from build123d import *

# Parameters (mm, degrees)
SKETCH1_R           = 87
SKETCH1_R_2         = 10
BOSS_EXTRUDE1_DEPTH = 5
SKETCH2_R           = 80
SKETCH2_R_2         = 76
BOSS_EXTRUDE2_DEPTH = 30
SKETCH3_R           = 87
SKETCH3_R_2         = 80
BOSS_EXTRUDE3_DEPTH = 20


with BuildPart() as part:
    # Sketch1 → Boss-Extrude1 (new body)
    with BuildSketch(Plane(origin=(0, 0, 0), x_dir=(1, 0, 0), z_dir=(0, 1, 0))):
        with Locations(Location((0, 0, 0), (0, 0, 270))):
            Circle(SKETCH1_R)
        with Locations(Location((0, 51.875, 0), (0, 0, 270))):
            Circle(SKETCH1_R_2, mode=Mode.SUBTRACT)
        with Locations(Location((44.926567821, -25.936633975, 0), (0, 0, 270))):
            Circle(SKETCH1_R_2, mode=Mode.SUBTRACT)
        with Locations(Location((-44.923567821, -25.938366025, 0), (0, 0, 270))):
            Circle(SKETCH1_R_2, mode=Mode.SUBTRACT)
    extrude(amount=BOSS_EXTRUDE1_DEPTH)

    # Sketch2 → Boss-Extrude2 (add)
    with BuildSketch(Plane(origin=(0, 5, 0), x_dir=(1, 0, 0), z_dir=(0, 1, 0))):
        with Locations(Location((0, 0, 0), (0, 0, 270))):
            Circle(SKETCH2_R)
        with Locations(Location((0, 0, 0), (0, 0, 270))):
            Circle(SKETCH2_R_2, mode=Mode.SUBTRACT)
    extrude(amount=BOSS_EXTRUDE2_DEPTH)

    # Sketch3 → Boss-Extrude3 (add)
    with BuildSketch(Plane(origin=(0, 5, 0), x_dir=(1, 0, 0), z_dir=(0, 1, 0))):
        with Locations(Location((0, 0, 0), (0, 0, 270))):
            Circle(SKETCH3_R)
        with Locations(Location((0, 0, 0), (0, 0, 270))):
            Circle(SKETCH3_R_2, mode=Mode.SUBTRACT)
    extrude(amount=BOSS_EXTRUDE3_DEPTH)


solid = part.part
Input: part model. Units: mm. Frame: model coordinates. A direction names the side the tool comes from. Round coordinates to 2 decimals unless told otherwise and drop trailing zeros. Order: outer loops, then holes, each group sorted by start corner. A loop starts at its lowest first (then second) coordinate and runs counter-clockwise, first axis right, second up. Notation, with made-up numbers: (14, -29) - (19, -29) arc R22 cw to (19, -21) - close; hole circle Ø8 at (9.5, 56). An arc over 180 degrees is marked (long way). Use a Markdown table: item, result.
1. Mould query, pull axis Z, two halves, no side actions, for faces 3 (the face through (-29, 35, 71)), 4 (the face through (-78.1, 29.93, -17.34)), 5 (the face through (36.055, 2.465, 30.551)). Classes: +Z half, -Z half, draft (parallel to the pull), parting line (faces both ways), or undercut.
Evaluation:
| item | result |
|---|---|
| face 3 | draft |
| face 4 | parting line |
| face 5 | undercut |
2. Material intervals for probe 1 along X at (y, z) = (23, -2.5); probe 2 along Z at (x, y) = (1.5, 28); probe 3 along Y at (x, z) = (70, 26), sorted ascending.
Evaluation:
| item | result |
|---|---|
| probe 1 | -86.96 to -75.96, 75.96 to 86.96 |
| probe 2 | -79.99 to -75.99, 75.99 to 79.99 |
| probe 3 | 0 to 5 |
3. Section B-B on z = 32. Return the cut outline in (x, y).
Evaluation:
| item | result |
|---|---|
| outline | (-80.9, 0) - (-52.88, 0) - (-52.88, 5) - (-68.93, 5) - (-68.93, 35) - (-73.32, 35) - (-73.32, 25) - (-80.9, 25) - close; (-36.97, 0) - (36.97, 0) - (36.97, 5) - (-36.97, 5) - close; (52.88, 0) - (80.9, 0) - (80.9, 25) - (73.32, 25) - (73.32, 35) - (68.93, 35) - (68.93, 5) - (52.88, 5) - close |
4. Section A-A on x = 0. Return the cut outline in (y, z) (3 decimals).
Evaluation:
| item | result |
|---|---|
| outline | (0, -87) - (25, -87) - (25, -80) - (35, -80) - (35, -76) - (5, -76) - (5, -61.875) - (0, -61.875) - close; (0, -41.875) - (5, -41.875) - (5, 76) - (35, 76) - (35, 80) - (25, 80) - (25, 87) - (0, 87) - close |
5. Section C-C on z = -59.5. Return the cut outline in (x, y), then the cut area to 3 significant figures.
Evaluation:
| item | result |
|---|---|
| outline | (-63.47, 0) - (-6.47, 0) - (-6.47, 5) - (-47.28, 5) - (-47.28, 35) - (-53.48, 35) - (-53.48, 25) - (-63.47, 25) - close; (6.47, 0) - (63.47, 0) - (63.47, 25) - (53.48, 25) - (53.48, 35) - (47.28, 35) - (47.28, 5) - (6.47, 5) - close |
| area | 1,340 mm^2 |
6. Access query for faces 1 (the face through (86.26, 12.32, -11.33)), 2 (the face through (1, 5, -1)). Directions: +Z, -Z, +X, -X, +Y, -Y. A direction counts if a zero-diameter tool reaches every point of the face in a straight line with its end or side. Return the directions, or none.
Evaluation:
| item | result |
|---|---|
| face 1 | +Y, -Y |
| face 2 | +Y |
7. Section D-D on y = 10.5. Return the cut outline in (x, z).
Evaluation:
| item | result |
|---|---|
| outline | circle Ø174 at (0, 0); hole circle Ø152 at (0, 0) |
8. First-contact query: pin 1 (16 mm diameter, centred on x = 44.93, z = 25.94, fed in from -Y); pin 2 (4 mm diameter, centred on y = 6.5, z = 38, fed in from +X); pin 3 (1 mm diameter, centred on y = 10, z = -35.5, fed in from -X); pin 4 (4 mm diameter, centred on y = 31.5, z = -25.5, fed in from -X). Flat tips, straight axial feed; report the tip coordinate or a pass-through.
Evaluation:
| item | result |
|---|---|
| pin 1 | through |
| pin 2 | x = 79.2 |
| pin 3 | x = -79.65 |
| pin 4 | x = -76.47 |
